```python
from build123d import *

# Parameters (mm, degrees)
CROQUIS1_W              = 1
CROQUIS1_H              = 3
SALIENTE_EXTRUIR1_DEPTH = 48
SALIENTE_EXTRUIR2_DEPTH = 3
CROQUIS3_W              = 38.5
CROQUIS3_H              = 90.5
CORTAR_EXTRUIR1_DEPTH   = 2.2
CORTAR_EXTRUIR2_DEPTH   = 2.9


with BuildPart() as part:
    # Croquis1 → Saliente-Extruir1 (new body)
    with BuildSketch(Plane.XY):
        with BuildLine():
            ThreePointArc((1.1, 120.1), (2.6, 121.6), (4.1, 120.1))
            Line((4.1, 120.1), (4.1, 0.1))
            Line((4.1, 0.1), (1.1, 0.1))
            Line((1.1, 0.1), (1.1, 120.1))
        make_face()
        with BuildLine():
            Line((1, 0), (1, -3))
            ThreePointArc((1, -3), (3.192031022, -2.092031022), (4.1, 0.1))
            Line((4.1, 0.1), (1.1, 0.1))
            ThreePointArc((1.1, 0.1), (1.070710678, 0.029289322), (1, 0))
        make_face()
        with Locations((0.5, -1.5)):
            Rectangle(CROQUIS1_W, CROQUIS1_H)
    extrude(amount=SALIENTE_EXTRUIR1_DEPTH)

    # Croquis2 → Saliente-Extruir2 (add)
    with BuildSketch(Plane(origin=(0, 0, 0), x_dir=(-1, 0, 0), z_dir=(0, 0, -1))):
        with BuildLine():
            Line((-1, -3), (0, -3))
            Line((0, -3), (0, 120.1))
            ThreePointArc((0, 120.1), (-0.439339828, 121.160660172), (-1.5, 121.6))
            Line((-1.5, 121.6), (-2.6, 121.6))
            ThreePointArc((-2.6, 121.6), (-3.660660172, 121.160660172), (-4.1, 120.1))
            Line((-4.1, 120.1), (-4.1, 0.1))
            ThreePointArc((-4.1, 0.1), (-3.192031022, -2.092031022), (-1, -3))
        make_face()
    extrude(amount=SALIENTE_EXTRUIR2_DEPTH)

    # Croquis3 → Cortar-Extruir1 (cut)
    with BuildSketch(Plane(origin=(4.1, 0, 0), x_dir=(0, 0, -1), z_dir=(1, 0, 0))):
        with Locations((-28.75, 76.35)):
            Rectangle(CROQUIS3_W, CROQUIS3_H)
    extrude(amount=-CORTAR_EXTRUIR1_DEPTH, mode=Mode.SUBTRACT)

    # Croquis4 → Cortar-Extruir2 (cut, through all)
    with BuildSketch(Plane(origin=(1.9, 0, 0), x_dir=(0, 0, -1), z_dir=(1, 0, 0))):
        with BuildLine():
            Line((-9.5, 120.6), (-9.5, 121.426649916))
            Line((-9.5, 121.426649916), (-48, 121.426649916))
            Line((-48, 121.426649916), (-48, 31.1))
            Line((-48, 31.1), (-47, 31.1))
            Line((-47, 31.1), (-47, 32.1))
            ThreePointArc((-47, 32.1), (-19.983171743, 72.73430247), (-10.5, 120.6))
            Line((-10.5, 120.6), (-9.5, 120.6))
        make_face()
    extrude(amount=-CORTAR_EXTRUIR2_DEPTH, mode=Mode.SUBTRACT)


solid = part.part
```
Design review of the part built by this model. Coordinates are the model's own, in mm. A direction names the side the tool comes from. Give positions to 0.01 mm unless a question says otherwise; leave off trailing zeros. Loops run counter-clockwise (first coordinate to the right, second up) from the corner with the lowest first, then second, coordinate; pieces in that order, holes last. Notation, with made-up numbers: M 58.5,17.5 L 64.5,17.5 A20 cw 64.5,32.5 Z; hole C 77,-4 d4. An arc over 180 degrees is marked long. Return JSON: item names as keys, results as strings. Group by question number.
Item 1: For probe 1 along X at (y, z) = (2, 18); probe 2 along Z at (x, y) = (0.4, 46), list the stretches that pass through material, from the lowest coordinate up.
Item 2: We need section B-B (z = 18.5). Give the boundary of the cut face in (x, y), and give its area (3 significant figures).
Item 3: We need section D-D (y = 98.5). Give the boundary of the cut face in (x, z).
Item 4: Tool access review of faces 1 (the flat face through (0.7, 61.7, 0)), 2 (the flat face through (3, 14, 48)), 3 (the flat face through (1.9, 53, 21)): name each direction out of +Z, -Z, +X, -X, +Y, -Y from which nothing blocks a thin tool from reaching the whole face with its end or side.
Item 5: We need section C-C (x = 3.45). Give the boundary of the cut face in (y, z).
Item 6: We need section A-A (y = 6). Give the boundary of the cut face in (x, z).
Item 7: Insertion check: pin 1 Ø10 at (y, z) = (66.5, 26) entering from -X; pin 2 Ø0.6 at (x, y) = (1.5, 121) entering from +Z; pin 3 Ø2 at (x, z) = (2, 30.5) entering from -Y; pin 4 Ø1 at (x, z) = (3.5, 13) entering from -Y. Each pin has a flat end and moves straight along its axis. Give the tip position at first contact, or say it passes through.
Output:
{
 "1": {"probe 1": "x = 1.1 to 4.1", "probe 2": "z = -3 to 0"},
 "2": {"outline": "M 0,-3 L 1,-3 A3.1 ccw 4.1,0.1 L 4.1,31.1 L 1.9,31.1 L 1.9,76.5 L 1.1,76.5 L 1.1,0.1 A0.1 cw 1,0 L 0,0 Z", "area": "140 mm^2"},
 "3": {"outline": "M 0,-3 L 4.1,-3 L 4.1,9.5 L 1.9,9.5 L 1.9,12.46 L 1.1,12.46 L 1.1,0 L 0,0 Z"},
 "4": {"face 1": "+Z, -X, +Y", "face 2": "+Z, +X, -X, +Y, -Y", "face 3": "+Z, +X, +Y"},
 "5": {"outline": "M -1.8,-3 L 121.34,-3 L 121.34,9.5 L 31.1,9.5 L 31.1,48 L -1.8,48 Z"},
 "6": {"outline": "M 0,-3 L 4.1,-3 L 4.1,48 L 1.1,48 L 1.1,0 L 0,0 Z"},
 "7": {"pin 1": "stops at x = 1.1", "pin 2": "stops at z = 9.5", "pin 3": "stops at y = -3", "pin 4": "stops at y = -2.27"}
}
